Geometry check sheet. Reference: the model listing, model coordinates, mm. A direction names the side the tool comes from. Round coordinates to 2 decimals unless told otherwise and drop trailing zeros. Write each loop counter-clockwise with the first axis right and the second up, starting at its lowest first coordinate (ties: lowest second). Pieces come first, ordered by that corner, then holes. Notation, with made-up numbers: (76.5, -4) - (111.5, -4) arc R11 cw to (111.5, 4) - close; hole circle Ø5 at (-28, 38). An arc over 180 degrees is marked (long way). Return JSON: item names as keys, results as strings.
```python
from build123d import *

# Parameters (mm, degrees)
EXTRUDE_1_DEPTH     = 19
CUT_EXTRUDE_1_DEPTH = 8
SKETCH_3_R          = 1.1
CUT_EXTRUDE_2_DEPTH = 8


with BuildPart() as part:
    # 草图1 → 凸台-拉伸1 (new body)
    with BuildSketch(Plane.XY):
        Polygon((-1.935, 3.351518313), (1.935, 3.351518313), (3.87, 0), (1.935, -3.351518313), (-1.935, -3.351518313), (-3.87, 0), align=None)
    extrude(amount=EXTRUDE_1_DEPTH)

    # 草图2 → 切除-拉伸1 (cut)
    with BuildSketch(Plane.XY.offset(19)):
        with BuildLine():
            Line((-1.118033989, 1), (1.118033989, 1))
            ThreePointArc((1.118033989, 1), (0, -1.5), (-1.118033989, 1))
        make_face()
    extrude(amount=-CUT_EXTRUDE_1_DEPTH, mode=Mode.SUBTRACT)

    # 草图3 → 切除-拉伸2 (cut)
    with BuildSketch(Plane(origin=(0, 0, 0), x_dir=(-1, 0, 0), z_dir=(0, 0, -1))):
        Circle(SKETCH_3_R)
    extrude(amount=-CUT_EXTRUDE_2_DEPTH, mode=Mode.SUBTRACT)


solid = part.part
```
(1) Access from +Z, -Z, +X, -X, +Y, -Y to the whole of each face (thin tool, end or side, straight path). Record for faces 1 (the face through (-1.05, 0.33, 3.94)), 2 (the face through (0, 0, 11)), 3 (the face through (-2.89, -1.7, 9.37)).
Response values:
{"face 1": "-Z", "face 2": "+Z", "face 3": "+Z, -Z, -X, -Y"}
(2) Section check B-B, the plane x = 0. Enter the section's corners in (y, z).
Response values:
{"outline": "(-3.35, 0) - (-1.1, 0) - (-1.1, 8) - (1.1, 8) - (1.1, 0) - (3.35, 0) - (3.35, 19) - (1, 19) - (1, 11) - (-1.5, 11) - (-1.5, 19) - (-3.35, 19) - close"}
(3) Material ranges on line 1 along Y through (x, z) = (1, 4); line 2 along Y through (x, z) = (0, 3.5); line 3 along X through (y, z) = (-2.75, 10.25), recorded low to high. Write a range as [from, to].
Response values:
{"line 1": "y = [-3.35, -0.46], [0.46, 3.35]", "line 2": "y = [-3.35, -1.1], [1.1, 3.35]", "line 3": "x = [-2.28, 2.28]"}
(4) Section check A-A, the plane z = 6.5. Enter the section's corners in (x, y) (3 decimals), plus the area to 3 significant figures.
Response values:
{"outline": "(-3.87, 0) - (-1.935, -3.352) - (1.935, -3.352) - (3.87, 0) - (1.935, 3.352) - (-1.935, 3.352) - close; hole circle Ø2.2 at (0, 0)", "area": "35.1 mm^2"}
(5) Release check for a two-part mould opening along Y. For faces 4 (the face through (0, 2, 19)), 5 (the face through (0, -3.352, 9)), 6 (the face through (0, -1.5, 15.1)) record: pulls with the +Y half, pulls with the -Y half, needs draft (parallel to the pull), parting line crosses it, or undercut.
Response values:
{"face 4": "needs draft", "face 5": "pulls with the -Y half", "face 6": "undercut"}
(6) Gauge pin test, flat ends, axial feed: pin 1 (2 mm diameter, centred on y = -2.5, z = 11, fed in from -X); pin 2 (3 mm diameter, centred on y = -2, z = 5.5, fed in from -X); pin 3 (2.5 mm diameter, centred on x = 0, y = 0, fed in from +Z); pin 4 (0.7 mm diameter, centred on x = 0, y = 0.5, fed in from -Z). Record the tip position at first contact, or that the pin passes through.
Response values:
{"pin 1": "stops at x = -3", "pin 2": "stops at x = -3.58", "pin 3": "stops at z = 19", "pin 4": "stops at z = 8"}
(7) Section check C-C, the plane z = 15.5. Enter the section's corners in (x, y) (3 decimals).
Response values:
{"outline": "(-3.87, 0) - (-1.935, -3.352) - (1.935, -3.352) - (3.87, 0) - (1.935, 3.352) - (-1.935, 3.352) - close; hole (-1.118, 1) arc R1.5 ccw (long way) to (1.118, 1) - close"}
(8) Section check D-D, the plane y = 0.25. Enter the section's corners in (x, z), plus the area to 3 significant figures.
Response values:
{"outline": "(-3.73, 0) - (-1.07, 0) - (-1.07, 8) - (1.07, 8) - (1.07, 0) - (3.73, 0) - (3.73, 19) - (1.48, 19) - (1.48, 11) - (-1.48, 11) - (-1.48, 19) - (-3.73, 19) - close", "area": "101 mm^2"}
